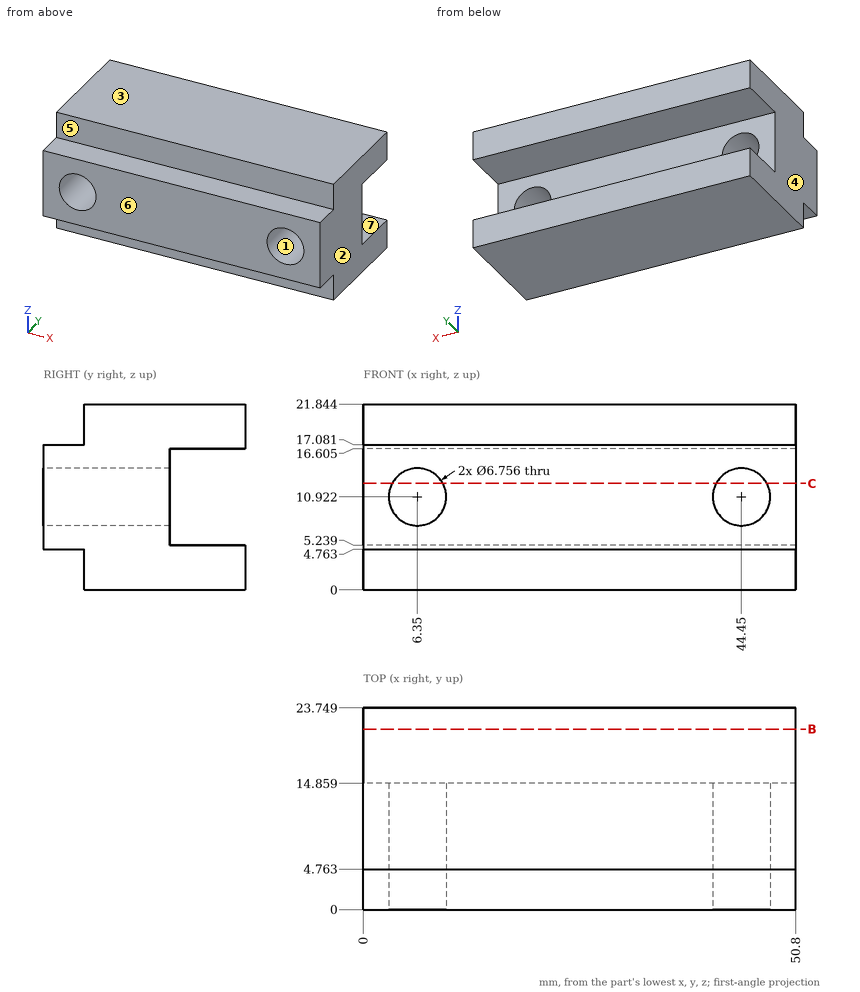
Input: dimensioned drawing with shaded views. Units: mm. Origin: part minimum x, y, z. A direction names the side the tool comes from. Give positions to 0.01 mm unless a question says otherwise; leave off trailing zeros. Loops run counter-clockwise (first coordinate to the right, second up) from the corner with the lowest first, then second, coordinate; pieces in that order, holes last. Notation, with made-up numbers: M -5.5,55.25 L 39.5,55.25 A15 ccw 39.5,74.25 Z; hole C 80,-15 d10. An arc over 180 degrees is marked long. Put each result on its own line as item: value.
1) Cut plane B-B, the plane y = 21.25. Return the cut outline in (x, z) (1 decimal), plus the area to 3 significant figures.
Computed values:
outline: M 0,0 L 50.8,0 L 50.8,5.2 L 0,5.2 Z; M 0,16.6 L 50.8,16.6 L 50.8,21.8 L 0,21.8 Z
area: 532 mm^2
2) Cut plane C-C, the plane z = 12.5. Return the cut outline in (x, y).
Computed values:
outline: M 0,0 L 3.36,0 L 3.36,14.86 L 0,14.86 Z; M 9.34,0 L 41.46,0 L 41.46,14.86 L 9.34,14.86 Z; M 47.44,0 L 50.8,0 L 50.8,14.86 L 47.44,14.86 Z
3) First-contact query: P1, Ø3.5, axis at x = 27, z = 11, coming from the +Y side; P2, Ø4, axis at x = 23.5, z = 1.5, coming from the -Y side; P3, Ø4, axis at x = 13.5, y = 2, coming from the -Z side; P4, Ø8, axis at y = 20.5, z = 10.5, coming from the -X side. Flat tips, straight axial feed; report the tip coordinate or a pass-through.
Computed values:
P1: stops at y = 14.86
P2: stops at y = 4.76
P3: stops at z = 4.76
P4: passes through
4) Material intervals for L1, parallel to Z at x = 42, y = 22.25 (1 decimal); L2, parallel to X at y = 14.5, z = 11.25; L3, parallel to Z at x = 44.45, y = 3.5, sorted ascending. Write a range as from..to.
Computed values:
L1: z = 0..5.2, 16.6..21.8
L2: x = 0..2.99, 9.71..41.09, 47.81..50.8
L3: z = 4.76..7.54, 14.3..17.08
5) Reachability of the marked faces 5, 6 and 7 from +Z, -Z, +X, -X, +Y, -Y: full face, straight path, thin tool, end or side. Return the list, or none.
Computed values:
face 5: +Z, +X, -X, -Y
face 6: +Z, -Z, +X, -X, -Y
face 7: +X, -X, +Y
6) Mould query, pull axis X, two halves, no side actions, for the marked faces 1, 2, 3 and 4. Classes: released by +X, released by -X, zero draft, split by the parting line, or undercut.
Computed values:
face 1: undercut
face 2: released by +X
face 3: zero draft
face 4: released by -X
